Check sheet for the drawn part. Datum: minimum x, y, z corner. Units: mm. A direction names the side the tool comes from. Round coordinates to 2 decimals unless told otherwise and drop trailing zeros. Write each loop counter-clockwise with the first axis right and the second up, starting at its lowest first coordinate (ties: lowest second). Pieces come first, ordered by that corner, then holes. Notation, with made-up numbers: (32, 69) -> (88, 69) arc R34 ccw to (88, 101) -> close; hole circle Ø8 at (30, 47.5). An arc over 180 degrees is marked (long way). Use a Markdown table: item, result.
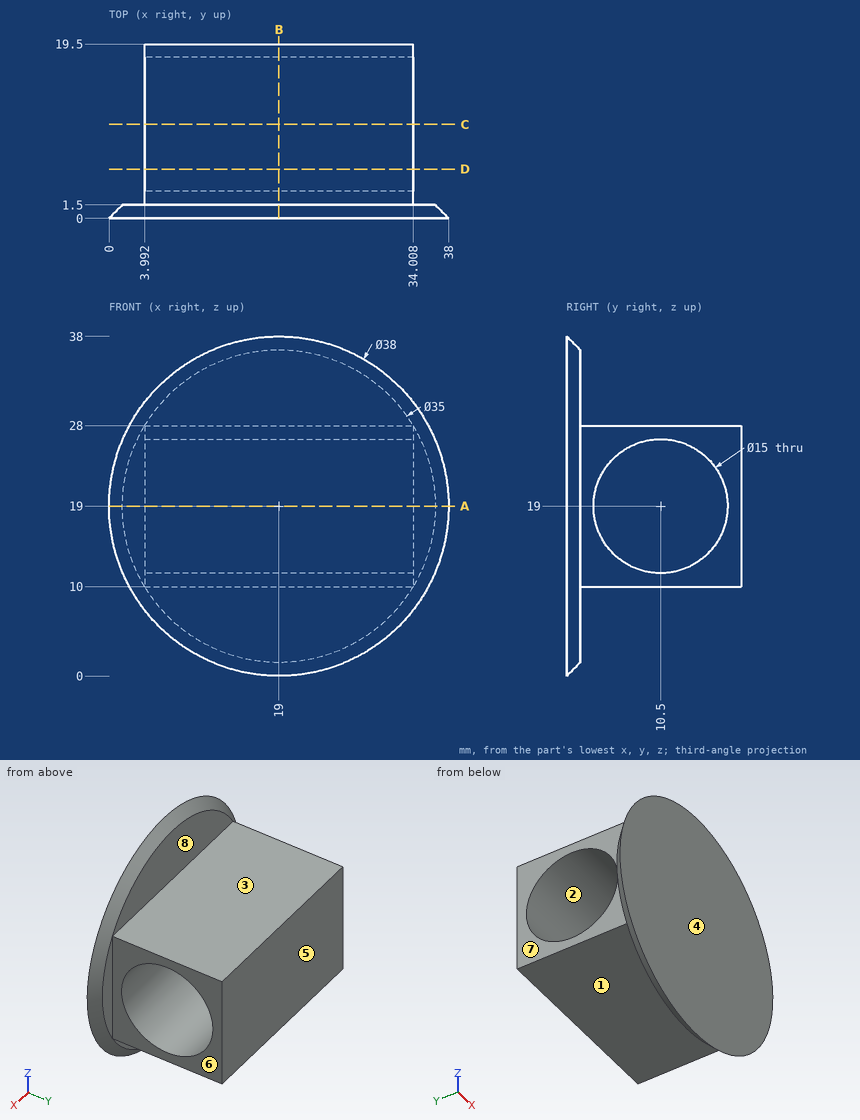
(1) Section check B-B on x = 19. Record the cut outline in (y, z), plus the area to 3 significant figures.
A:
| item | result |
|---|---|
| outline | (0, 0) -> (1.5, 1.5) -> (1.5, 10) -> (19.5, 10) -> (19.5, 28) -> (1.5, 28) -> (1.5, 36.5) -> (0, 38) -> close; hole circle Ø15 at (10.5, 19) |
| area | 202 mm2 |
(2) Section check A-A on z = 19. Record the cut outline in (x, y), plus the area to 3 significant figures.
A:
| item | result |
|---|---|
| outline | (0, 0) -> (38, 0) -> (36.5, 1.5) -> (34.01, 1.5) -> (34.01, 3) -> (3.99, 3) -> (3.99, 1.5) -> (1.5, 1.5) -> close; (3.99, 18) -> (34.01, 18) -> (34.01, 19.5) -> (3.99, 19.5) -> close |
| area | 145 mm2 |
(3) Gauge pin test, flat ends, axial feed: pin 1 Ø7 at (x, z) = (21.5, 4) entering from +Y; pin 2 Ø9 at (x, y) = (23, 9) entering from +Z; pin 3 Ø5 at (y, z) = (5.5, 29.5) entering from +X. Record the tip position at first contact, or that the pin passes through.
A:
| item | result |
|---|---|
| pin 1 | stops at y = 1.5 |
| pin 2 | stops at z = 28 |
| pin 3 | stops at x = 34.01 |
(4) Section check C-C on y = 10.5. Record the cut outline in (x, z).
A:
| item | result |
|---|---|
| outline | (3.99, 10) -> (34.01, 10) -> (34.01, 11.5) -> (3.99, 11.5) -> close; (3.99, 26.5) -> (34.01, 26.5) -> (34.01, 28) -> (3.99, 28) -> close |
(5) Release check for a two-part mould opening along Z. For the marked faces 1, 2 and 3 record: +Z half, -Z half, draft (parallel to the pull), parting line (faces both ways), or undercut.
A:
| item | result |
|---|---|
| face 1 | -Z half |
| face 2 | undercut |
| face 3 | +Z half |
(6) Section check D-D on y = 5.5. Record the cut outline in (x, z).
A:
| item | result |
|---|---|
| outline | (3.99, 10) -> (34.01, 10) -> (34.01, 13.41) -> (3.99, 13.41) -> close; (3.99, 24.59) -> (34.01, 24.59) -> (34.01, 28) -> (3.99, 28) -> close |
(7) Access from +Z, -Z, +X, -X, +Y, -Y to the whole of each face (thin tool, end or side, straight path). Record for the marked faces 4, 5, 6, 7 and 8.
A:
| item | result |
|---|---|
| face 4 | +Z, -Z, +X, -X, -Y |
| face 5 | +Z, -Z, +X, -X, +Y |
| face 6 | +Z, -Z, +X, +Y |
| face 7 | +Z, -Z, -X, +Y |
| face 8 | +Z, +X, -X, +Y |
(8) Thickness scan on line 1 (Y direction, x = 21.5, z = 19); line 2 (Y direction, x = 29, z = 6); line 3 (X direction, y = 2, z = 25). Record the ranges inside material, lowest first.
A:
| item | result |
|---|---|
| line 1 | y = 0 to 3, 18 to 19.5 |
| line 2 | y = 0 to 1.5 |
| line 3 | x = 3.99 to 34.01 |
